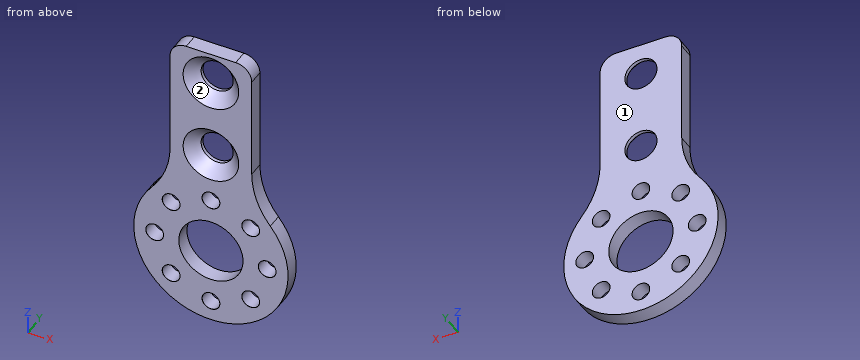
from build123d import *

# Parameters (mm, degrees)
BOSS_EXTRUDE1_DEPTH                            = 4.7625
M5_CLEARANCE_HOLE1_D                           = 5.5
M5_CLEARANCE_HOLE1_CSINK_D                     = 5.55
M5_CLEARANCE_HOLE1_CSINK_ANGLE                 = 90
SKETCH5_R                                      = 10
CUT_EXTRUDE1_DEPTH                             = 73.611133199
CSK_FOR_M8_FLAT_HEAD_MACHINE_SCREW1_AT_2_COUNT = 2
CSK_FOR_M8_FLAT_HEAD_MACHINE_SCREW1_AT_2_PITCH = 25
FILLET1_R                                      = 25
FILLET2_R                                      = 5


with BuildPart() as part:
    # Sketch1 → Boss-Extrude1 (new body)
    with BuildSketch(Plane(origin=(0, 0, 0), x_dir=(1, 0, 0), z_dir=(0, 1, 0))):
        with BuildLine():
            Line((-12.7, -68.364429774), (12.7, -68.364429774))
            Line((12.7, -68.364429774), (12.7, -20.364429774))
            ThreePointArc((12.7, -20.364429774), (0, 24), (-12.7, -20.364429774))
            Line((-12.7, -20.364429774), (-12.7, -68.364429774))
        make_face()
    extrude(amount=BOSS_EXTRUDE1_DEPTH)

    # M5 Clearance Hole1 (through all)
    with Locations(Plane(origin=(0, 0, 0), x_dir=(-1, 0, 0), z_dir=(0, -1, 0))):
        with Locations((0, 17.5), (12.374368671, 12.374368671), (17.5, 0), (12.374368671, -12.374368671), (0, -17.5), (-12.374368671, -12.374368671), (-17.5, 0), (-12.374368671, 12.374368671)):
            CounterSinkHole(M5_CLEARANCE_HOLE1_D / 2, M5_CLEARANCE_HOLE1_CSINK_D / 2, counter_sink_angle=M5_CLEARANCE_HOLE1_CSINK_ANGLE)

    # Sketch5 → Cut-Extrude1 (cut, through all)
    with BuildSketch(Plane.XZ):
        with Locations(Location((0, 0, 0), (0, 0, 270))):
            Circle(SKETCH5_R)
    extrude(amount=-CUT_EXTRUDE1_DEPTH, mode=Mode.SUBTRACT)

    # Sketch8 → CSK for M8 Flat Head Machine Screw1 (revolve, cut)
    with BuildSketch(Plane(origin=(0, 0, 33.364429774), x_dir=(0, 0, -1), z_dir=(1, 0, 0))):
        Polygon((0, 0), (0, 4.7625), (5, 4.7625), (5, 3.65), (8.65, 0), align=None)
    csk_for_m8_flat_head_machine_screw1 = revolve(axis=Axis((0, -6.35, 33.364429774), (0, 1, 0)), mode=Mode.SUBTRACT)

    # CSK for M8 Flat Head Machine Screw1 at 2: CSK for M8 Flat Head Machine Screw1 ×2
    with Locations(*[(0, 0, i * CSK_FOR_M8_FLAT_HEAD_MACHINE_SCREW1_AT_2_PITCH) for i in range(1, CSK_FOR_M8_FLAT_HEAD_MACHINE_SCREW1_AT_2_COUNT)]):
        add(csk_for_m8_flat_head_machine_screw1, mode=Mode.SUBTRACT)

    # Fillet1
    fillet1_edges = [part.edges().sort_by_distance(p)[0] for p in [
        (-12.7, 2.38125, 20.364429774),
        (12.7, 2.38125, 20.364429774),
    ]]
    fillet(fillet1_edges, radius=FILLET1_R)

    # Fillet2
    fillet2_edges = [part.edges().sort_by_distance(p)[0] for p in [
        (12.7, 2.38125, 68.364429774),
        (-12.7, 2.38125, 68.364429774),
    ]]
    fillet(fillet2_edges, radius=FILLET2_R)


solid = part.part
Read the model definition and answer for the solid it produces. Units are mm, in the model's axes. Face numbers are marked on the shaded views. Give positions to 0.01 mm unless a question says otherwise; leave off trailing zeros. Loops run counter-clockwise (first coordinate to the right, second up) from the corner with the lowest first, then second, coordinate; pieces in that order, holes last. Notation, with made-up numbers: (8, 29.25) - (25, 29.25) arc R10 ccw to (25, 38.25) - close; hole circle Ø3 at (23, 59). An arc over 180 degrees is marked (long way). Answer as CSV lines item,"result". Start each with the question number.
1) Find section A-A (x = 0). State how many separate pieces and enclosed holes the cut face has, then the cut area to 3 significant figures.
2) Each of these flat-tipped pins is pushed along its axis until it touches: pin 1 Ø16 at (x, z) = (0, 33.36) entering from +Y; pin 2 Ø4.5 at (x, z) = (-12.37, -12.37) entering from +Y (3 decimals); pin 3 Ø11.5 at (x, z) = (0, 58.36) entering from -Y; pin 4 Ø2.5 at (y, z) = (3, 51.5) entering from +X. Where does it stop, or does it pass through?
3) Determine the mould class of the marked faces 1 and 2 for opening direction X: released by +X, released by -X, zero draft, split by the parting line, or undercut.
4) Find section B-B (z = -7.5). Write down the section's boundary in (x, y), then the cut area to 3 significant figures.
5) Straight lines are drawn through the part: L1, parallel to Z at x = -14.5, y = 2.1; L2, parallel to Z at x = 5, y = 0.85; L3, parallel to X at y = 1.6, z = 9. For each, find the intervals that lie inside material, in ascending order. Write a range as from..to.
Findings below:
1,separate pieces,"6"
1,enclosed holes,"0"
1,area,"170 mm^2"
2,pin 1,"y = 4.76"
2,pin 2,"through"
2,pin 3,"y = 2.9"
2,pin 4,"x = 12.7"
3,face 1,"zero draft"
3,face 2,"undercut"
4,outline,"(-22.8, 0) - (-6.61, 0) - (-6.61, 4.76) - (-22.8, 4.76) - close; (6.61, 0) - (22.8, 0) - (22.8, 4.76) - (6.61, 4.76) - close"
4,area,"154 mm^2"
5,L1,"-19.12..-14.12, -10.63..10.63, 14.12..21.99"
5,L2,"-23.47..-8.66, 8.66..27.38, 39.35..52.38, 64.35..68.36"
5,L3,"-22.25..-4.36, 4.36..22.25"
